The listing builds one solid part. Answer for the finished solid, in the listing's coordinates (mm). Face numbers are marked on the shaded views. A direction names the side the tool comes from. Round coordinates to 2 decimals unless told otherwise and drop trailing zeros. Use a Markdown table: item, result. Add a question column.
1) A tool of negligible diameter and unlimited length cuts with its end or side. For the marked faces 1 and 2, from which of +Z, -Z, +X, -X, +Y, -Y can it reach the whole face along a straight path? Write none if from no direction.
2) Find the intervals of material crossed by probe 1 along Z at (x, y) = (0.5, 0); probe 2 along Y at (x, z) = (6.75, 0); probe 3 along Y at (x, z) = (12.95, 0), in increasing order. Write a range as from..to.
3) Each of these flat-tipped pins is pushed along its axis until it touches: P1, Ø4, axis at x = -0.5, z = -3.5, coming from the -Y side; P2, Ø4, axis at x = -2.5, y = -2, coming from the -Z side; P3, Ø6, axis at y = 0, z = 0, coming from the -X side; P4, Ø8, axis at y = 0, z = 1, coming from the -X side. Where does it stop, or does it pass through?
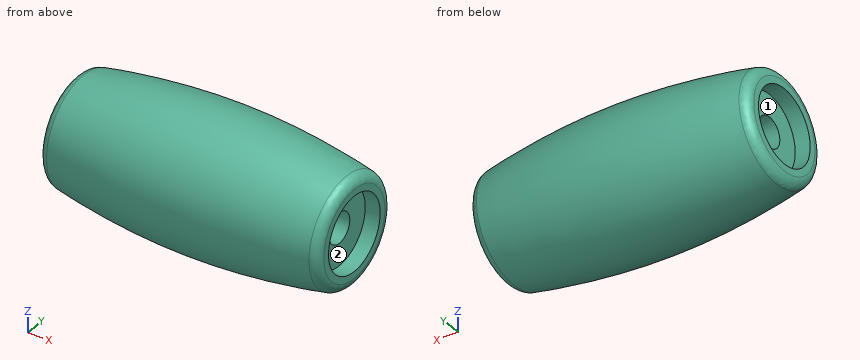
Autodesk Inventor part; units mm, degrees
ref_plane "YZ Plane" through (0, 0, 0) normal (1, 0, 0) x (0, 1, 0)
ref_plane "XZ Plane" through (0, 0, 0) normal (0, 1, 0) x (-1, 0, 0)
ref_plane "XY Plane" through (0, 0, 0) normal (0, 0, 1) x (1, 0, 0)
sketch "Sketch1" plane through (0, 0, 0) normal (0, 1, 0) x (-1, 0, 0)
  line L0 (0, 0) -> (-14, 0)
  line L1 (0, 0) -> (14, 0)
  line L2 (-14, 0) -> (-14, -5.25)
  line L3 (14, 0) -> (14, -5.25)
  arc A0 (-14, -5.25) -> (14, -5.25) centre (0, 61.6112) ccw
  line L4 (0, -6.7) -> (0, 0) construction
  dimension "d0" = 14
  dimension "d1" = 14
  dimension "d2" = 5.25
  dimension "d3" = 6.7
revolve "Revolution1" add sketch "Sketch1" angle 360 about axis through (0, 0, 0) along (-1, 0, 0)
fillet "Fillet1" radius 1 2 edges at (14, 0, 5.25) (-14, 0, 5.25)
sketch "Sketch2" plane through (-14, 0, 0) normal (-1, 0, 0) x (0, 0, 1)
  circle A0 centre (0, 0) radius 3.75
  dimension "d6" = 7.5
extrude "Extrusion1" cut sketch "Sketch2" against normal blind 1.5
mirror "Mirror1" about plane through (0, 0, 0) normal (1, 0, 0) of "Extrusion1"
sketch "Sketch3" plane through (12.5, 0, 0) normal (1, 0, 0) x (0, 0, -1)
  circle A0 centre (0, 0) radius 3.75
hole "Hole1" at (12.5, 0, 0) direction (-1, 0, 0) diameter 3.015 end through all
properties part number "roller" material "Rubber, Black"
Entries:
| question | item | result |
|---|---|---|
| 1 | face 1 | -X |
| 1 | face 2 | +X |
| 2 | probe 1 | z = -6.7..-1.51, 1.51..6.7 |
| 2 | probe 2 | y = -6.37..-1.51, 1.51..6.37 |
| 2 | probe 3 | y = -5.46..-3.75, 3.75..5.46 |
| 3 | P1 | stops at y = -6.53 |
| 3 | P2 | stops at z = -6.68 |
| 3 | P3 | stops at x = -12.5 |
| 3 | P4 | stops at x = -14 |
